Can you work these out from the model? Positions are in its coordinate system, mm. Give positions to 0.01 mm unless a question says otherwise; leave off trailing zeros.
from build123d import *

# Parameters (mm, degrees)
SKETCH_1_W          = 390
SKETCH_1_H          = 270
EXTRUDE_1_DEPTH     = 4
FILLET_1_R          = 40
SKETCH_2_R          = 3.25
CUT_EXTRUDE_1_DEPTH = 238.204553076


with BuildPart() as part:
    # 草图1 → 凸台-拉伸1 (new body)
    with BuildSketch(Plane(origin=(0, 0, 0), x_dir=(1, 0, 0), z_dir=(0, 1, 0))):
        Rectangle(SKETCH_1_W, SKETCH_1_H)
    extrude(amount=EXTRUDE_1_DEPTH)

    # 圆角1
    fillet_1_edges = [part.edges().sort_by_distance(p)[0] for p in [
        (195, 2, 135),
        (-195, 2, 135),
        (-195, 2, -135),
        (195, 2, -135),
    ]]
    fillet(fillet_1_edges, radius=FILLET_1_R)

    # 草图2 → 切除-拉伸1 (cut, through all)
    with BuildSketch(Plane(origin=(0, 4, 0), x_dir=(1, 0, 0), z_dir=(0, 1, 0))):
        with Locations(Location((-185, -77, 0), (0, 0, 270))):
            Circle(SKETCH_2_R)
        with Locations(Location((-185, 77, 0), (0, 0, 270))):
            Circle(SKETCH_2_R)
        with Locations(Location((-90, 125, 0), (0, 0, 270))):
            Circle(SKETCH_2_R)
        with Locations(Location((-90, -125, 0), (0, 0, 270))):
            Circle(SKETCH_2_R)
        with Locations(Location((90, -125, 0), (0, 0, 270))):
            Circle(SKETCH_2_R)
        with Locations(Location((185, -77, 0), (0, 0, 270))):
            Circle(SKETCH_2_R)
        with Locations(Location((185, 77, 0), (0, 0, 270))):
            Circle(SKETCH_2_R)
        with Locations(Location((90, 125, 0), (0, 0, 270))):
            Circle(SKETCH_2_R)
    extrude(amount=-CUT_EXTRUDE_1_DEPTH, mode=Mode.SUBTRACT)


solid = part.part
(1) Will these pins go through, and if not, where does the flat tip stop? P1, Ø4, axis at x = 185, z = -77, coming from the -Y side; P2, Ø1, axis at y = 2, z = -107.5, coming from the -X side.
Returned:
P1: passes through
P2: stops at x = -193.16
(2) Imagine slicing it at A-A, the plane y = 3.25. Give the number of separate pieces and of enclosed holes in the cut face, plus the area to 3 significant figures.
Returned:
separate pieces: 1
enclosed holes: 8
area: 104,000 mm2
(3) If I drill on L1, parallel to X at y = 1.4, z = 77; L2, parallel to Z at x = 185, y = 3.05; L3, parallel to X at y = 0.9, z = -76, over which ranges is the centre line in solid material (lowest first)?
Returned:
L1: x = -195 to -188.25, -181.75 to 181.75, 188.25 to 195
L2: z = -121.46 to -80.25, -73.75 to 73.75, 80.25 to 121.46
L3: x = -195 to -188.09, -181.91 to 181.91, 188.09 to 195
